Geometry check sheet. Reference: the model listing, model coordinates, mm. Face numbers are marked on the shaded views. A direction names the side the tool comes from. Coordinates: 2 decimals unless noted, no trailing zeros. Order: outer loops, then holes, each group sorted by start corner. A loop starts at its lowest first (then second) coordinate and runs counter-clockwise, first axis right, second up. Notation, with made-up numbers: (-28.5, 70) - (-13.5, 70) arc R21 ccw to (-13.5, 83) - close; hole circle Ø9 at (-23.75, -34). An arc over 180 degrees is marked (long way). Use CSV: the item, a comma, the result in double quotes. Start each with the question number.
1) Sectioned sample at B-B, the plane x = 36.65. Record the cut outline in (y, z).
2) Sectioned sample at D-D, the plane y = -16.5. Record the cut outline in (x, z), and give its area (3 significant figures).
3) Thickness scan on probe 1 along Y at (x, z) = (36.65, 1.25); probe 2 along X at (y, z) = (-36, 4); probe 3 along Z at (x, y) = (5.5, -3). Record the ranges inside material, lowest first. Write a range as [from, to].
4) Tool access check on the marked faces 1 and 2. Record the directions out of +Z, -Z, +X, -X, +Y, -Y that give a thin tool (end or side, any length) a straight path to the whole face; none if there is none.
5) Sectioned sample at C-C, the plane x = 21.15. Record the cut outline in (y, z).
6) Depth check by flat-ended pin: P1, Ø19.5, axis at y = -18, z = -21, coming from the +X side; P2, Ø3, axis at x = 5.5, y = -37, coming from the +Z side; P3, Ø4, axis at x = 36.65, y = -36.65, coming from the -Z side. Enter the tip coordinate at first touch or a pass-through.
7) Sectioned sample at A-A, the plane y = -36.65. Record the cut outline in (x, z), and give its area (3 significant figures).
8) Draft check along Y on the marked faces 3, 4, 5 and 6. Enter one of: released by +Y, released by -Y, zero draft, split by the parting line, or undercut.
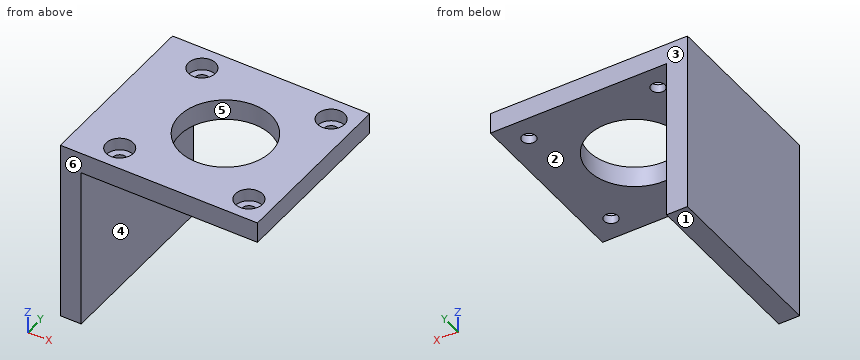
from build123d import *

# Parameters (mm, degrees)
F1_DEPTH       = 42.3
F3_D           = 3.3
F3_DEPTH       = 10
F3_CBORE_D     = 6.5
F3_CBORE_DEPTH = 3
F3_TIP         = 0.9914200214
F4_D           = 22


with BuildPart() as f1:
    # F0 (on Front) → F1 (new body)
    with BuildSketch(Plane.XZ):
        Polygon((0, -39), (0, 0), (42.3, 0), (42.3, 5), (-5, 5), (-5, -39), align=None)
    extrude(amount=F1_DEPTH)

    # F3
    with Locations(Plane.XY.offset(5)):
        with Locations((5.65, -5.65), (36.65, -5.65), (36.65, -36.65), (5.65, -36.65)):
            CounterBoreHole(F3_D / 2, F3_CBORE_D / 2, F3_CBORE_DEPTH, depth=F3_DEPTH)
            with Locations((0, 0, -(F3_DEPTH + F3_TIP / 2))):  # 118° drill point
                Cone(0, F3_D / 2, F3_TIP, mode=Mode.SUBTRACT)

    # F4 (through all)
    with Locations(Plane.XY.offset(5)):
        with Locations((21.15, -21.15)):
            Hole(F4_D / 2)


solid = f1.part
Evaluation:
1,outline,"(-42.3, 0) - (-38.3, 0) - (-38.3, 2) - (-39.9, 2) - (-39.9, 5) - (-42.3, 5) - close; (-35, 0) - (-7.3, 0) - (-7.3, 2) - (-8.9, 2) - (-8.9, 5) - (-33.4, 5) - (-33.4, 2) - (-35, 2) - close; (-4, 0) - (0, 0) - (0, 5) - (-2.4, 5) - (-2.4, 2) - (-4, 2) - close"
2,outline,"(-5, -39) - (0, -39) - (0, 0) - (11.18, 0) - (11.18, 5) - (-5, 5) - close; (31.12, 0) - (42.3, 0) - (42.3, 5) - (31.12, 5) - close"
2,area,"332 mm²"
3,probe 1,"[-42.3, -38.3], [-35, -7.3], [-4, 0]"
3,probe 2,"[-5, 2.47], [8.83, 33.47], [39.83, 42.3]"
3,probe 3,"[0, 2]"
4,face 1,"-Z, +X, -X, +Y, -Y"
4,face 2,"-Z, +X, +Y, -Y"
5,outline,"(-42.3, 0) - (-32.15, 0) - (-32.15, 5) - (-42.3, 5) - close; (-10.15, 0) - (0, 0) - (0, 5) - (-10.15, 5) - close"
6,P1,"x = 0"
6,P2,"z = 2"
6,P3,"z = 0"
7,outline,"(-5, -39) - (0, -39) - (0, 0) - (4, 0) - (4, 2) - (2.4, 2) - (2.4, 5) - (-5, 5) - close; (7.3, 0) - (35, 0) - (35, 2) - (33.4, 2) - (33.4, 5) - (8.9, 5) - (8.9, 2) - (7.3, 2) - close; (38.3, 0) - (42.3, 0) - (42.3, 5) - (39.9, 5) - (39.9, 2) - (38.3, 2) - close"
7,area,"379 mm²"
8,face 3,"released by +Y"
8,face 4,"zero draft"
8,face 5,"undercut"
8,face 6,"released by -Y"
